The listing builds one solid part. Answer for the finished solid, in the listing's coordinates (mm). Coordinates: 2 decimals unless noted, no trailing zeros. Loops run counter-clockwise (first coordinate to the right, second up) from the corner with the lowest first, then second, coordinate; pieces in that order, holes last. Notation, with made-up numbers: M -5.75,54 L 18.25,54 A13 ccw 18.25,78 Z; hole C 21,-3 d10. An arc over 180 degrees is marked long. Return JSON: item names as keys, results as strings. Group by question number.
1. Section A-A (z = -39) is taken. Write down the section's boundary in (x, y).
2. Straight lines are drawn through the part: L1, parallel to X at y = 0.4, z = -10; L2, parallel to X at y = 1.05, z = -25; L3, parallel to X at y = 0.5, z = -30. For each, find the intervals that lie inside material, in ascending order. Write a range as from..to.
3. Section D-D (y = 0.9) is taken. Count the separate pieces of the cut face and the enclosed holes in it, then the cut area to 3 significant figures.
4. Section C-C (x = -23.5) is taken. Write down the section's boundary in (y, z), then the cut area to 3 significant figures.
5. Given P1, Ø0.8, axis at y = 0.5, z = -112.5, coming from the -X side; P2, Ø0.8, axis at y = 1, z = -80, coming from the +X side, each flat-ended and moving along its own axis, determine where each tip first touches the part or whether it passes through.
6. Section B-B (x = 42) is taken. Write down the section's boundary in (y, z), then the cut area to 3 significant figures.
7. The mould has two halves that part along Z. Classify faces 1 (the face through (42.07, 0.74, -101.7)), 2 (the face through (1, 1.5, -61)), 3 (the face through (17.83, 0.74, -11.27)): pulls with the +Z half, pulls with the -Z half, needs draft (parallel to the pull), parting line crosses it, or undercut.
```python
from build123d import *

# Parameters (mm, degrees)
SKETCH1_R           = 1.1
SKETCH1_R_2         = 1.7
SKETCH1_R_3         = 1.6
SKETCH1_W           = 50
SKETCH1_H           = 10
SKETCH1_W_2         = 15
SKETCH1_H_2         = 2.5
SKETCH1_W_3         = 5
SKETCH1_H_3         = 50
BOSS_EXTRUDE1_DEPTH = 1.5


with BuildPart() as part:
    # Sketch1 → Boss-Extrude1 (new body)
    with BuildSketch(Plane(origin=(0, 0, 0), x_dir=(1, 0, 0), z_dir=(0, 1, 0))):
        Polygon((-45, 105), (-50.5, 105), (-50.5, 120), (50.5, 120), (50.5, 105), (45, 105), (45, 70), (55, 70), (55, 50), (45, 50), (45, 0), (-45, 0), (-45, 50), (-55, 50), (-55, 70), (-45, 70), align=None)
        with Locations(Location((48, 110.5, 0), (0, 0, 270))):
            Circle(SKETCH1_R, mode=Mode.SUBTRACT)
        with Locations(Location((-48, 110.5, 0), (0, 0, 270))):
            Circle(SKETCH1_R, mode=Mode.SUBTRACT)
        with Locations(Location((42, 100, 0), (0, 0, 270))):
            Circle(SKETCH1_R_2, mode=Mode.SUBTRACT)
        with Locations(Location((-42, 100, 0), (0, 0, 270))):
            Circle(SKETCH1_R_2, mode=Mode.SUBTRACT)
        with Locations(Location((-42, 25, 0), (0, 0, 270))):
            Circle(SKETCH1_R_2, mode=Mode.SUBTRACT)
        with Locations(Location((42, 25, 0), (0, 0, 270))):
            Circle(SKETCH1_R_2, mode=Mode.SUBTRACT)
        with Locations(Location((-18.8, 10, 0), (0, 0, 270))):
            Circle(SKETCH1_R_3, mode=Mode.SUBTRACT)
        with Locations(Location((18.8, 10, 0), (0, 0, 270))):
            Circle(SKETCH1_R_3, mode=Mode.SUBTRACT)
        with Locations((0, 112.5)):
            Rectangle(SKETCH1_W, SKETCH1_H, mode=Mode.SUBTRACT)
        with Locations((-44.5, 67)):
            Rectangle(SKETCH1_W_2, SKETCH1_H_2, mode=Mode.SUBTRACT)
        with Locations((-44.5, 53)):
            Rectangle(SKETCH1_W_2, SKETCH1_H_2, mode=Mode.SUBTRACT)
        with Locations((44.5, 53)):
            Rectangle(SKETCH1_W_2, SKETCH1_H_2, mode=Mode.SUBTRACT)
        with Locations((17.5, 45)):
            Rectangle(SKETCH1_W_3, SKETCH1_H_3, mode=Mode.SUBTRACT)
        with Locations((-17.5, 45)):
            Rectangle(SKETCH1_W_3, SKETCH1_H_3, mode=Mode.SUBTRACT)
        with Locations((44.5, 67)):
            Rectangle(SKETCH1_W_2, SKETCH1_H_2, mode=Mode.SUBTRACT)
    extrude(amount=BOSS_EXTRUDE1_DEPTH)


solid = part.part
```
Worked out:
{
 "1": {"outline": "M -45,0 L -20,0 L -20,1.5 L -45,1.5 Z; M -15,0 L 15,0 L 15,1.5 L -15,1.5 Z; M 20,0 L 45,0 L 45,1.5 L 20,1.5 Z"},
 "2": {"L1": "-45..-20.4, -17.2..17.2, 20.4..45", "L2": "-45..-43.7, -40.3..-20, -15..15, 20..40.3, 43.7..45", "L3": "-45..-20, -15..15, 20..45"},
 "3": {"separate pieces": "1", "enclosed holes": "15", "area": "10,200 mm^2"},
 "4": {"outline": "M 0,-120 L 1.5,-120 L 1.5,-117.5 L 0,-117.5 Z; M 0,-107.5 L 1.5,-107.5 L 1.5,0 L 0,0 Z", "area": "165 mm^2"},
 "5": {"P1": "x = -50.5", "P2": "x = 45"},
 "6": {"outline": "M 0,-120 L 1.5,-120 L 1.5,-101.7 L 0,-101.7 Z; M 0,-98.3 L 1.5,-98.3 L 1.5,-68.25 L 0,-68.25 Z; M 0,-65.75 L 1.5,-65.75 L 1.5,-54.25 L 0,-54.25 Z; M 0,-51.75 L 1.5,-51.75 L 1.5,-26.7 L 0,-26.7 Z; M 0,-23.3 L 1.5,-23.3 L 1.5,0 L 0,0 Z", "area": "162 mm^2"},
 "7": {"face 1": "undercut", "face 2": "needs draft", "face 3": "undercut"}
}
